Job drawing, mm, ordinate dimensions from the low corner. One solid piece. A direction names the side the tool comes from. Give positions to 0.01 mm unless a question says otherwise; leave off trailing zeros. Write each loop counter-clockwise with the first axis right and the second up, starting at its lowest first coordinate (ties: lowest second). Pieces come first, ordered by that corner, then holes. Notation, with made-up numbers: (3, -26) -> (49, -26) arc R30 ccw to (49, 10) -> close; hole circle Ø3 at (57.5, 9.25). An arc over 180 degrees is marked (long way). One line per question, with ' | ' between items. Start each with the question number.
(1) Band-saw the part on B-B, the plane x = 5. Give the cut face in (y, z), and give its area (3 significant figures).
(2) Tool access for the marked faces 1 and 2: list every direction of +Z, -Z, +X, -X, +Y, -Y with a clear straight run to the whole face (end or side of a thin tool).
(3) Drill centre lines: probe 1 along X at (y, z) = (18.5, 5.25); probe 2 along Z at (x, y) = (5, 1.25); probe 3 along X at (y, z) = (27.5, 5) (1 decimal). Where is each one in solid material? Low to high. Write a range as from..to.
(4) Band-saw the part on C-C, the plane z = 9.25. Give the cut face in (x, y).
(5) Band-saw the part on A-A, the plane y = 17.5. Give the cut face in (x, z).
(6) Band-saw the part on D-D, the plane x = 29. Give the cut face in (y, z), and give its area (3 significant figures).
(7) Pin check, flat tips, straight feed: P1, Ø5, axis at y = 9, z = 3.5, coming from the +X side; P2, Ø5, axis at x = 4, z = 4.5, coming from the +Y side; P3, Ø5, axis at y = 10.5, z = 6.5, coming from the -X side. Stop position of each tip, or through.
(8) Pull direction X, two halves, no side cores. Call the marked faces 3, 4, 5 and 6: released by +X, released by -X, zero draft, split by the parting line, or undercut.
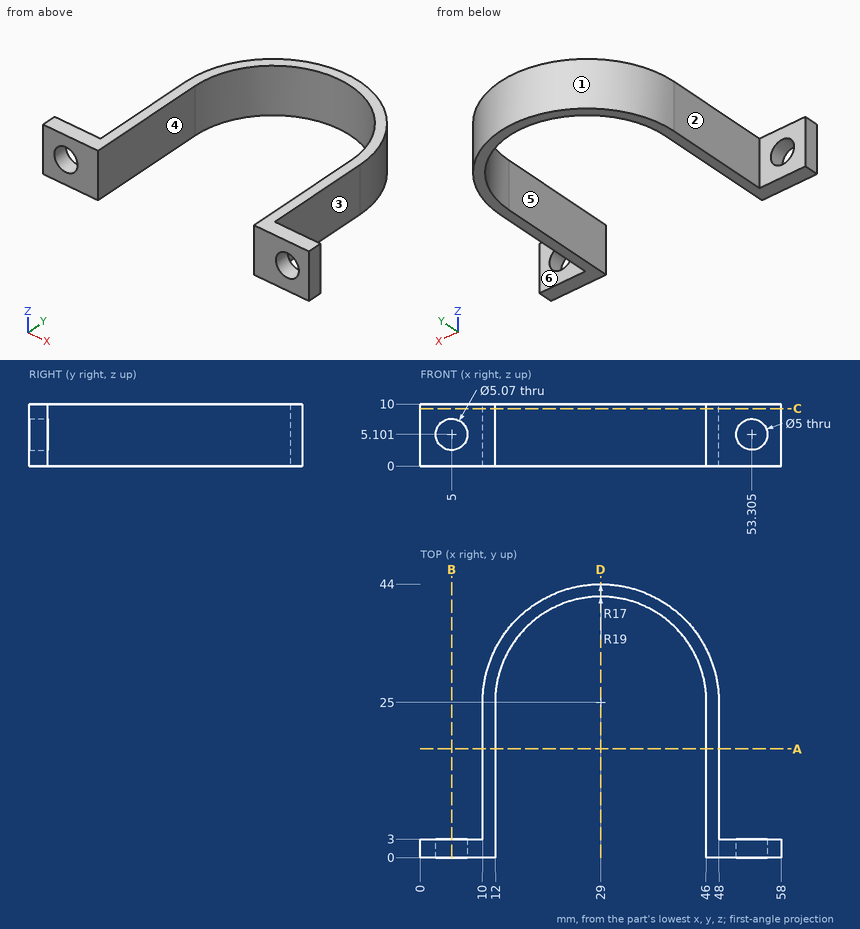
Results:
1) outline: (0, 0) -> (3, 0) -> (3, 2.57) -> (0, 2.57) -> close; (0, 7.64) -> (3, 7.64) -> (3, 10) -> (0, 10) -> close | area: 14.8 mm²
2) face 1: +Z, -Z, +Y | face 2: +Z, -Z, -X, +Y
3) probe 1: x = 10..12, 46..48 | probe 2: z = 0..2.57, 7.64..10 | probe 3: x = 10.2..12.2, 45.8..47.8
4) outline: (0, 0) -> (12, 0) -> (12, 25) arc R17 cw to (46, 25) -> (46, 0) -> (58, 0) -> (58, 3) -> (48, 3) -> (48, 25) arc R19 ccw to (10, 25) -> (10, 3) -> (0, 3) -> close
5) outline: (10, 0) -> (12, 0) -> (12, 10) -> (10, 10) -> close; (46, 0) -> (48, 0) -> (48, 10) -> (46, 10) -> close
6) outline: (42, 0) -> (44, 0) -> (44, 10) -> (42, 10) -> close | area: 20.0 mm²
7) P1: stops at x = 48 | P2: stops at y = 3 | P3: stops at x = 10
8) face 3: released by +X | face 4: undercut | face 5: undercut | face 6: zero draft
